Verification items for the finished model (mm, model axes). A direction names the side the tool comes from. Give positions to 0.01 mm unless a question says otherwise; leave off trailing zeros. Write each loop counter-clockwise with the first axis right and the second up, starting at its lowest first coordinate (ties: lowest second). Pieces come first, ordered by that corner, then holes. Notation, with made-up numbers: (16, 28.25) - (40, 28.25) arc R13 ccw to (40, 32.25) - close; hole circle Ø3 at (26, 35). An arc over 180 degrees is marked (long way). Answer as a JSON object with one key per item and string values. Group by question number.
Item 1: Sectioned sample at C-C, the plane y = 31.5. Record the boundary of the cut face in (x, z), and give its area (3 significant figures).
Item 2: Sectioned sample at D-D, the plane x = 0. Record the boundary of the cut face in (y, z).
Item 3: Sectioned sample at A-A, the plane z = 14. Record the boundary of the cut face in (x, y).
Item 4: Scan lines: line 1 along X through (y, z) = (6, -10); line 2 along X through (y, z) = (3.5, -2); line 3 along Y through (x, z) = (6, 2). Record each from-to range of solid material in increasing order. Write a range as [from, to].
Item 5: Go/stop test with flat-tipped pins: pin 1 (2 mm diameter, centred on x = 2.5, z = -12.5, fed in from +Y); pin 2 (10 mm diameter, centred on x = 15, y = 30.5, fed in from -Z); pin 3 (12 mm diameter, centred on x = -13.5, y = 43.5, fed in from +Z); pin 4 (3 mm diameter, centred on y = 24.5, z = -14.5, fed in from -X). Record where each tip stops, or that it passes through.
Item 6: Sectioned sample at B-B, the plane x = -10. Record the boundary of the cut face in (y, z).
Item 7: Draft check along Z on faces 4 (the face through (0, 4, -20)), 5 (the face through (11.5, 3.9, 10.9)), 6 (the face through (19, 50, 14)). Enter one of: +Z half, -Z half, draft (parallel to the pull), parting line (faces both ways), or undercut.
Item 8: Tool access check on faces 1 (the face through (-19, 50, 14)), 2 (the face through (-17.31, 28.71, -15.84)), 3 (the face through (0, 4, 15)). Record the directions out of +Z, -Z, +X, -X, +Y, -Y that give a thin tool (end or side, any length) a straight path to the whole face; none if there is none.
```python
from build123d import *

# Parameters (mm, degrees)
SKETCH1_W            = 50
SKETCH1_H            = 40
SKETCH1_R            = 2.5
SKETCH1_R_2          = 1.75
MAIN_STRUCTURE_DEPTH = 8
SKETCH1_3_R          = 2.5
BOSS_EXTRUDE2_DEPTH  = 3
SKETCH1_4_R          = 2.5
SHAFTS_DEPTH         = 50


with BuildPart() as part:
    # Sketch1 → Main Structure (new body)
    with BuildSketch(Plane(origin=(0, 0, 0), x_dir=(1, 0, 0), z_dir=(0, 1, 0))):
        Rectangle(SKETCH1_W, SKETCH1_H)
        with Locations(Location((-19, 14, 0), (0, 0, 270))):
            Circle(SKETCH1_R, mode=Mode.SUBTRACT)
        with Locations(Location((-19, -14, 0), (0, 0, 90))):
            Circle(SKETCH1_R, mode=Mode.SUBTRACT)
        with Locations(Location((19, 14, 0), (0, 0, 90))):
            Circle(SKETCH1_R, mode=Mode.SUBTRACT)
        with Locations(Location((19, -14, 0), (0, 0, 270))):
            Circle(SKETCH1_R, mode=Mode.SUBTRACT)
        with Locations(Location((-10, 10, 0), (0, 0, 270))):
            Circle(SKETCH1_R_2, mode=Mode.SUBTRACT)
        with Locations(Location((-10, -10, 0), (0, 0, 90))):
            Circle(SKETCH1_R_2, mode=Mode.SUBTRACT)
        with Locations(Location((10, -10, 0), (0, 0, 270))):
            Circle(SKETCH1_R_2, mode=Mode.SUBTRACT)
        with Locations(Location((10, 10, 0), (0, 0, 90))):
            Circle(SKETCH1_R_2, mode=Mode.SUBTRACT)
        with BuildLine():
            Line((-14, 7.5), (-14, -7.5))
            ThreePointArc((-14, -7.5), (-16, -9.5), (-18, -7.5))
            Line((-18, -7.5), (-18, 7.5))
            ThreePointArc((-18, 7.5), (-16, 9.5), (-14, 7.5))
        make_face(mode=Mode.SUBTRACT)
        with BuildLine():
            Line((14, 7.5), (14, -7.5))
            ThreePointArc((14, -7.5), (16, -9.5), (18, -7.5))
            Line((18, -7.5), (18, 7.5))
            ThreePointArc((18, 7.5), (16, 9.5), (14, 7.5))
        make_face(mode=Mode.SUBTRACT)
        with BuildLine():
            Line((5, 10), (5, -10))
            ThreePointArc((5, -10), (0, -15), (-5, -10))
            Line((-5, -10), (-5, 10))
            ThreePointArc((-5, 10), (0, 15), (5, 10))
        make_face(mode=Mode.SUBTRACT)
    extrude(amount=MAIN_STRUCTURE_DEPTH)

    # Sketch1_3 → Boss-Extrude2 (add)
    with BuildSketch(Plane(origin=(0, 0, 0), x_dir=(1, 0, 0), z_dir=(0, 1, 0))):
        with Locations(Location((-19, 14, 0), (0, 0, 270))):
            Circle(SKETCH1_3_R)
        with Locations(Location((19, 14, 0), (0, 0, 90))):
            Circle(SKETCH1_3_R)
        with Locations(Location((-19, -14, 0), (0, 0, 90))):
            Circle(SKETCH1_3_R)
        with Locations(Location((19, -14, 0), (0, 0, 270))):
            Circle(SKETCH1_3_R)
    extrude(amount=BOSS_EXTRUDE2_DEPTH)

    # Sketch1_4 → Shafts (add)
    with BuildSketch(Plane(origin=(0, 0, 0), x_dir=(1, 0, 0), z_dir=(0, 1, 0))):
        with Locations(Location((-19, -14, 0), (0, 0, 90))):
            Circle(SKETCH1_4_R)
        with Locations(Location((19, -14, 0), (0, 0, 270))):
            Circle(SKETCH1_4_R)
        with Locations(Location((19, 14, 0), (0, 0, 90))):
            Circle(SKETCH1_4_R)
        with Locations(Location((-19, 14, 0), (0, 0, 270))):
            Circle(SKETCH1_4_R)
    extrude(amount=SHAFTS_DEPTH)


solid = part.part
```
Geometry check:
{
 "1": {"outline": "circle Ø5 at (-19, -14); circle Ø5 at (-19, 14); circle Ø5 at (19, -14); circle Ø5 at (19, 14)", "area": "78.5 mm^2"},
 "2": {"outline": "(0, -20) - (8, -20) - (8, -15) - (0, -15) - close; (0, 15) - (8, 15) - (8, 20) - (0, 20) - close"},
 "3": {"outline": "(-25, 0) - (-3, 0) - (-3, 8) - (-16.5, 8) - (-16.5, 50) - (-21.5, 50) - (-21.5, 8) - (-25, 8) - close; (3, 0) - (25, 0) - (25, 8) - (21.5, 8) - (21.5, 50) - (16.5, 50) - (16.5, 8) - (3, 8) - close"},
 "4": {"line 1": "[-25, -11.75], [-8.25, -5], [5, 8.25], [11.75, 25]", "line 2": "[-25, -18], [-14, -5], [5, 14], [18, 25]", "line 3": "[0, 8]"},
 "5": {"pin 1": "through", "pin 2": "z = -16.5", "pin 3": "z = 16.5", "pin 4": "x = -21.5"},
 "6": {"outline": "(0, -20) - (8, -20) - (8, -11.75) - (0, -11.75) - close; (0, -8.25) - (8, -8.25) - (8, 8.25) - (0, 8.25) - close; (0, 11.75) - (8, 11.75) - (8, 20) - (0, 20) - close"},
 "7": {"face 4": "-Z half", "face 5": "undercut", "face 6": "draft"},
 "8": {"face 1": "+Z, -Z, +X, -X, +Y", "face 2": "+Y", "face 3": "+Y, -Y"}
}
